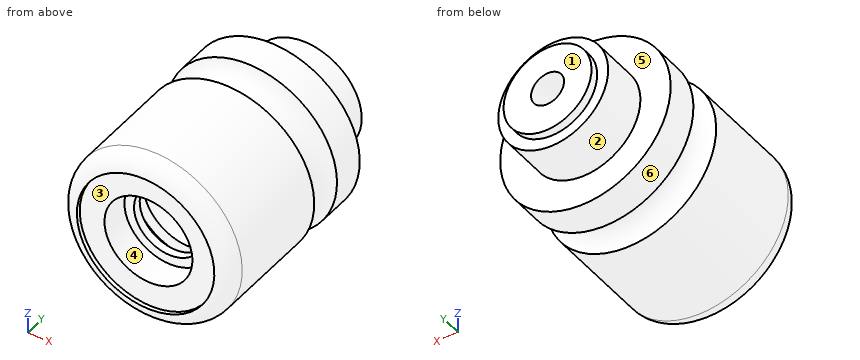
```python
from build123d import *


with BuildPart() as f1:
    # F0 (on Right) → F1 (revolve)
    with BuildSketch(Plane.YZ):
        with BuildLine():
            Line((44, 31), (6, 31))
            ThreePointArc((6, 31), (1.757359, 29.242641), (0, 25))
            Line((0, 25), (1.5, 25))
            Line((1.5, 25), (1.5, 16))
            Line((1.5, 16), (12, 16))
            Line((12, 16), (12, 12.5))
            Line((12, 12.5), (15, 12.5))
            Line((15, 12.5), (15, 20.5))
            Line((15, 20.5), (22, 20.5))
            Line((22, 20.5), (22, 16))
            Line((22, 16), (30, 16))
            Line((30, 16), (30, 6))
            Line((30, 6), (88, 6))
            Line((88, 6), (88, 16))
            Line((88, 16), (85, 16))
            Line((85, 16), (85, 20))
            Line((85, 20), (68, 20))
            Line((68, 20), (68, 31))
            Line((68, 31), (56, 31))
            ThreePointArc((56, 31), (50, 24.974378), (44, 31))
        make_face()
    revolve(axis=Axis((0, 44, 0), (0, 1, 0)))


solid = f1.part
```
The model under review builds one solid part; all positions refer to its coordinate system, in mm. Face numbers are marked on the shaded views. A direction names the side the tool comes from. Round coordinates to 2 decimals unless told otherwise and drop trailing zeros. Loops run counter-clockwise (first coordinate to the right, second up) from the corner with the lowest first, then second, coordinate; pieces in that order, holes last. Notation, with made-up numbers: (2.25, -4.5) -> (26.25, -4.5) arc R15 ccw to (26.25, 18.5) -> close; hole circle Ø5 at (12.5, -38). An arc over 180 degrees is marked (long way). Answer in a Markdown table with one row per item.
1) Draft analysis for pull direction X (two halves, no side actions). For the marked faces 4, 5 and 6, state which applies: pulls with the +X half, pulls with the -X half, needs draft (parallel to the pull), parting line crosses it, or undercut.
Taken from the geometry:
| item | result |
|---|---|
| face 4 | undercut |
| face 5 | needs draft |
| face 6 | parting line crosses it |
2) Consider section B-B, the plane y = 77.5. Write out the cut boundary in (x, z).
Taken from the geometry:
| item | result |
|---|---|
| outline | circle Ø40 at (0, 0); hole circle Ø12 at (0, 0) |
3) Wall thickness on line 1 along Y through (x, z) = (-3, -14.5); line 2 along Y through (x, z) = (18, 0); line 3 along X through (y, z) = (70, 0): over which ranges is each line inside the solid? List them lowest first.
Taken from the geometry:
| item | result |
|---|---|
| line 1 | y = 12 to 15, 30 to 88 |
| line 2 | y = 1.5 to 15, 22 to 85 |
| line 3 | x = -20 to -6, 6 to 20 |
4) Tool access review of the marked faces 1, 2 and 3: name each direction out of +Z, -Z, +X, -X, +Y, -Y from which nothing blocks a thin tool from reaching the whole face with its end or side.
Taken from the geometry:
| item | result |
|---|---|
| face 1 | +Z, -Z, +X, -X, +Y |
| face 2 | +Y |
| face 3 | -Y |
5) Consider section A-A, the plane y = 10.5. Write out the cut boundary in (x, z).
Taken from the geometry:
| item | result |
|---|---|
| outline | circle Ø62 at (0, 0); hole circle Ø32 at (0, 0) |
6) For pin 1 Ø20 at (x, z) = (0, 0) entering from -Y; pin 2 Ø2 at (x, y) = (-3, 37) entering from -Z; pin 3 Ø4 at (y, z) = (53.5, 9.5) entering from +X, all flat-tipped, find the tip position at first contact; note any pin that passes through.
Taken from the geometry:
| item | result |
|---|---|
| pin 1 | stops at y = 30 |
| pin 2 | stops at z = -30.94 |
| pin 3 | stops at x = 27 |
